```python
from build123d import *

# Parameters (mm, degrees)
BOSS_EXTRUDE1_DEPTH = 18
SKETCH2_W           = 200
SKETCH2_H           = 97
CUT_EXTRUDE1_DEPTH  = 19
CUT_EXTRUDE2_DEPTH  = 10


with BuildPart() as part:
    # Sketch1 → Boss-Extrude1 (new body)
    with BuildSketch(Plane.XY):
        with BuildLine():
            Line((0, 0), (51.303021499, -140.953893118))
            Line((51.303021499, -140.953893118), (-5.078535748, -161.475101717))
            ThreePointArc((-5.078535748, -161.475101717), (-59.282744504, -247.94612641), (-59.866905015, -350))
            Line((-59.866905015, -350), (-458.18031046, -350))
            ThreePointArc((-458.18031046, -350), (-530.476755656, -161.257646224), (-729.936822659, -193.909350133))
            ThreePointArc((-729.936822659, -193.909350133), (-786.401902791, -197.329105332), (-789.82165799, -140.864025199))
            ThreePointArc((-789.82165799, -140.864025199), (-684.665051265, -71.855170989), (-559.047216388, -65.507458149))
            ThreePointArc((-559.047216388, -65.507458149), (-324.287619955, -82.844559906), (-93.969262079, -34.202014333))
            Line((-93.969262079, -34.202014333), (0, 0))
        make_face()
    extrude(amount=BOSS_EXTRUDE1_DEPTH)

    # Sketch2 → Cut-Extrude1 (cut, through all)
    with BuildSketch(Plane.XY.offset(18)):
        with Locations((-187.508312236, -266.5)):
            Rectangle(SKETCH2_W, SKETCH2_H)
        with BuildLine():
            Line((-322.508312236, -315), (-432.508312236, -315))
            Line((-432.508312236, -315), (-432.508312236, -255))
            ThreePointArc((-432.508312236, -255), (-377.508312236, -200), (-322.508312236, -255))
            Line((-322.508312236, -255), (-322.508312236, -315))
        make_face()
    extrude(amount=-CUT_EXTRUDE1_DEPTH, mode=Mode.SUBTRACT)

    # Sketch3 → Cut-Extrude2 (cut)
    with BuildSketch(Plane.XY.offset(18)):
        Polygon((-1.01570715, -32.295020343), (29.76610575, -116.867356214), (-4.062828599, -129.180081374), (-34.844641498, -44.607745503), align=None)
    extrude(amount=-CUT_EXTRUDE2_DEPTH, mode=Mode.SUBTRACT)


solid = part.part
```
The model under review builds one solid part; all positions refer to its coordinate system, in mm. A direction names the side the tool comes from. Round coordinates to 2 decimals unless told otherwise and drop trailing zeros. Order: outer loops, then holes, each group sorted by start corner. A loop starts at its lowest first (then second) coordinate and runs counter-clockwise, first axis right, second up. Notation, with made-up numbers: M 29,53.25 L 35,53.25 A24 ccw 35,75.25 Z; hole C 43.5,-30 d4. An arc over 180 degrees is marked long. Use a Markdown table: item, result.
1) Consider section D-D (x = -604). Write out the cut boundary in (y, z), then the cut area to 3 significant figures.
Report:
| item | result |
|---|---|
| outline | M -140.12,0 L -60.08,0 L -60.08,18 L -140.12,18 Z |
| area | 1,440 mm^2 |
2) Consider section C-C (y = -302). Write out the cut boundary in (x, z), then the cut area to 3 significant figures.
Report:
| item | result |
|---|---|
| outline | M -450.18,0 L -432.51,0 L -432.51,18 L -450.18,18 Z; M -322.51,0 L -287.51,0 L -287.51,18 L -322.51,18 Z; M -87.51,0 L -66.68,0 L -66.68,18 L -87.51,18 Z |
| area | 1,320 mm^2 |
3) Consider section A-A (x = -398). Write out the cut boundary in (y, z), then the cut area to 3 significant figures.
Report:
| item | result |
|---|---|
| outline | M -350,0 L -315,0 L -315,18 L -350,18 Z; M -203.96,0 L -84.56,0 L -84.56,18 L -203.96,18 Z |
| area | 2,780 mm^2 |
4) Insertion check: pin 1 (1 mm diameter, centred on x = -585.5, z = 7.5, fed in from +Y); pin 2 (5.5 mm diameter, centred on y = -279.5, z = 6.5, fed in from -X); pin 3 (5.5 mm diameter, centred on y = -273, z = 11.5, fed in from -X). Each pin has a flat end and moves straight along its axis. Give the tip position at first contact, or say it passes through.
Report:
| item | result |
|---|---|
| pin 1 | y = -61.22 |
| pin 2 | x = -451.87 |
| pin 3 | x = -452.96 |
5) Consider section B-B (z = 13). Write out the cut boundary in (x, y), then the cut area to 3 significant figures.
Report:
| item | result |
|---|---|
| outline | M -789.82,-140.86 A40 ccw -729.94,-193.91 A160 cw -458.18,-350 L -59.87,-350 A186.53 cw -5.08,-161.48 L 51.3,-140.95 L 0,0 L -93.97,-34.2 A837.95 cw -559.05,-65.51 A240 ccw Z; hole M -432.51,-315 L -322.51,-315 L -322.51,-255 A55 ccw -432.51,-255 Z; hole M -287.51,-315 L -87.51,-315 L -87.51,-218 L -287.51,-218 Z; hole M -34.84,-44.61 L -4.06,-129.18 L 29.77,-116.87 L -1.02,-32.3 Z |
| area | 124,000 mm^2 |
6) Tool access review of faces 4 (the face through (-2, -80, 8)), 5 (the face through (23.51, -151.07, 8.87)), 6 (the face through (-378.718, -200.013, 9.126)): name each direction out of +Z, -Z, +X, -X, +Y, -Y from which nothing blocks a thin tool from reaching the whole face with its end or side.
Report:
| item | result |
|---|---|
| face 4 | +Z |
| face 5 | +Z, -Z, +X, -Y |
| face 6 | +Z, -Z |
7) Wall thickness on line 1 along X through (y, z) = (-244.5, 10.5); line 2 along X through (y, z) = (-283, 5.75); line 3 along X through (y, z) = (-211, 12.5): over which ranges is each line inside the solid? List them lowest first. Write a range as [from, to].
Report:
| item | result |
|---|---|
| line 1 | [-460.1, -431.5], [-323.52, -287.51], [-87.51, -58.25] |
| line 2 | [-451.07, -432.51], [-322.51, -287.51], [-87.51, -65.92] |
| line 3 | [-477.2, -410.51], [-344.51, -44.09] |
8) Draft analysis for pull direction X (two halves, no side actions). For faces 1 (the face through (-47.64, -17.34, 8.87)), 2 (the face through (-327.59, -83.06, 8.87)), 3 (the face through (-274, -173, 18)), state which applies: released by +X, released by -X, zero draft, split by the parting line, or undercut.
Report:
| item | result |
|---|---|
| face 1 | released by -X |
| face 2 | undercut |
| face 3 | zero draft |
